CAD build for the part. Positions are in the model's coordinates, mm. Face numbers are marked on the shaded views. Give positions to 0.01 mm unless a question says otherwise; leave off trailing zeros. Write each loop counter-clockwise with the first axis right and the second up, starting at its lowest first coordinate (ties: lowest second). Pieces come first, ordered by that corner, then holes. Notation, with made-up numbers: (16.5, -8) - (39.5, -8) arc R22 ccw to (39.5, 27) - close; hole circle Ø8 at (76.5, 1.25). An arc over 180 degrees is marked (long way). Put each result on its own line as item: value. Start each with the question number.
1. Cut at C-C on z = -80. List the corners of the cut face in (x, y).
2. Cut at D-D on y = 13. List the corners of the cut face in (x, z).
3. Wall check: line 1 (X direction, y = 4.5, z = 0); line 2 (X direction, y = 15.75, z = 0); line 3 (Y direction, x = 43.5, z = 56). Give the ranges that are in metal, low to high.
4. Drop flat-ended pins along their axis: pin 1 (18 mm diameter, centred on x = -80, z = 0, fed in from +Y); pin 2 (4 mm diameter, centred on x = -2, y = -5, fed in from +Z); pin 3 (12 mm diameter, centred on y = -1, z = 71, fed in from +X); pin 4 (6 mm diameter, centred on x = 66.5, y = 8.5, fed in from -Z). Give the stop position or say it passes through.
5. Cut at A-A on x = 0. List the corners of the cut face in (y, z).
6. Mould opens along Z. For the marked faces 1, 2 and 3 say: +Z half, -Z half, draft (parallel to the pull), parting line (faces both ways), or undercut.
7. Cut at B-B on y = -4.5. List the corners of the cut face in (x, z).
from build123d import *

# Parameters (mm, degrees)
SKETCH1_R           = 95
BOSS_EXTRUDE1_DEPTH = 10
SKETCH2_R           = 65
BOSS_EXTRUDE2_DEPTH = 10
SKETCH3_R           = 57.5
CUT_EXTRUDE1_DEPTH  = 10
SKETCH4_R           = 7
CUT_EXTRUDE2_DEPTH  = 136.830777072


with BuildPart() as part:
    # Sketch1 → Boss-Extrude1 (new, symmetric)
    with BuildSketch(Plane(origin=(0, 0, 0), x_dir=(1, 0, 0), z_dir=(0, 1, 0))):
        with Locations(Location((0, 0, 0), (0, 0, 270))):
            Circle(SKETCH1_R)
    extrude(amount=BOSS_EXTRUDE1_DEPTH, both=True)

    # Sketch2 → Boss-Extrude2 (add)
    with BuildSketch(Plane(origin=(0, 10, 0), x_dir=(1, 0, 0), z_dir=(0, 1, 0))):
        with Locations(Location((0, 0, 0), (0, 0, 270))):
            Circle(SKETCH2_R)
    extrude(amount=BOSS_EXTRUDE2_DEPTH)

    # Sketch3 → Cut-Extrude1 (cut)
    with BuildSketch(Plane(origin=(0, 20, 0), x_dir=(1, 0, 0), z_dir=(0, 1, 0))):
        with Locations(Location((0, 0, 0), (0, 0, 270))):
            Circle(SKETCH3_R)
    extrude(amount=-CUT_EXTRUDE1_DEPTH, mode=Mode.SUBTRACT)

    # Sketch4 → Cut-Extrude2 (cut, through all)
    with BuildSketch(Plane(origin=(0, 10, 0), x_dir=(1, 0, 0), z_dir=(0, 1, 0))):
        with Locations(Location((0, 80, 0), (0, 0, 270))):
            Circle(SKETCH4_R)
        with Locations(Location((80, 0, 0), (0, 0, 270))):
            Circle(SKETCH4_R)
        with Locations(Location((0, -80, 0), (0, 0, 270))):
            Circle(SKETCH4_R)
        with Locations(Location((-80, 0, 0), (0, 0, 270))):
            Circle(SKETCH4_R)
    extrude(amount=-CUT_EXTRUDE2_DEPTH, mode=Mode.SUBTRACT)


solid = part.part
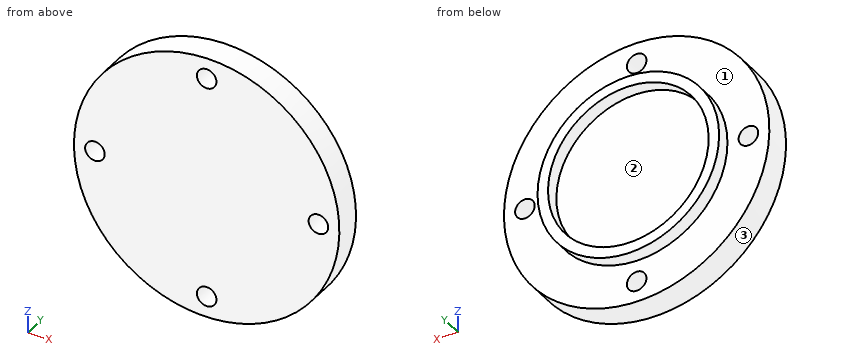
Report:
1. outline: (-51.23, -10) - (-7, -10) - (-7, 10) - (-51.23, 10) - close; (7, -10) - (51.23, -10) - (51.23, 10) - (7, 10) - close
2. outline: circle Ø130 at (0, 0); hole circle Ø115 at (0, 0)
3. line 1: x = -95 to -87, -73 to 73, 87 to 95
3. line 2: x = -65 to -57.5, 57.5 to 65
3. line 3: y = -10 to 10
4. pin 1: stops at y = 10
4. pin 2: stops at z = 95
4. pin 3: stops at x = 69.28
4. pin 4: stops at z = -70.66
5. outline: (-10, -95) - (10, -95) - (10, -87) - (-10, -87) - close; (-10, -73) - (10, -73) - (10, -65) - (20, -65) - (20, -57.5) - (10, -57.5) - (10, 57.5) - (20, 57.5) - (20, 65) - (10, 65) - (10, 73) - (-10, 73) - close; (-10, 87) - (10, 87) - (10, 95) - (-10, 95) - close
6. face 1: draft
6. face 2: undercut
6. face 3: parting line
7. outline: circle Ø190 at (0, 0); hole circle Ø14 at (-80, 0); hole circle Ø14 at (0, -80); hole circle Ø14 at (0, 80); hole circle Ø14 at (80, 0)
